Design review of the part built by this model. Coordinates are the model's own, in mm. A direction names the side the tool comes from. Round coordinates to 2 decimals unless told otherwise and drop trailing zeros. Order: outer loops, then holes, each group sorted by start corner. A loop starts at its lowest first (then second) coordinate and runs counter-clockwise, first axis right, second up. Notation, with made-up numbers: M -6.75,-39.75 L 29.25,-39.75 A19 ccw 29.25,-11.75 Z; hole C -21,14.25 d2. An arc over 180 degrees is marked long. Write each question's results on one line, items separated by ' | '. Start each with the question number.
Item 1: Take a section at A-A, the plane z = 0. Write out the cut boundary in (x, y), plus the area to 3 significant figures.
Item 2: Wall thickness on line 1 (X direction, y = -40.5, z = 6); line 2 (Z direction, x = 15, y = 37); line 3 (Y direction, x = 151, z = -5): over which ranges is each line inside the solid? List them lowest first. Write a range as [from, to].
Item 3: Machinability: for faces 1 (the flat face through (22, 42.2, 0.1)), 2 (the flat face through (74, 11, 7.5)), 3 (the flat face through (187, -11, -11)), 4 (the flat face through (107.186, 13.474, 0.105)), which of the approach directions +Z, -Z, +X, -X, +Y, -Y give a long, thin tool a straight path to every point of the face, cutting with its end or side? Answer none if there is none.
Item 4: Take a section at C-C, the plane x = 148.5. Write out the cut boundary in (y, z), plus the area to 3 significant figures.
Item 5: Take a section at B-B, the plane y = 0. Write out the cut boundary in (x, z), plus the area to 3 significant figures.
Item 6: Clearance check with flat-ended pins moving along their axes: pin 1 (4 mm diameter, centred on y = -5, z = 0, fed in from +X); pin 2 (4 mm diameter, centred on x = 56, z = -3, fed in from -Y); pin 3 (9 mm diameter, centred on y = 37, z = 0, fed in from -X); pin 4 (1 mm diameter, centred on x = 123.5, z = -4.5, fed in from -Y). State where each tip first meets the part, or that it passes through.
Item 7: The part is to be moulded in two halves that separate along Y. For faces 5 (the flat face through (22, -41, 3.4)), 6 (the cylindrical face through (195.163, -6.128, 0.154)), 7 (the flat face through (104.692, -8.598, 0.105)), 8 (the flat face through (104.692, 8.598, 0.105)), say which applies: +Y half, -Y half, draft (parallel to the pull), parting line (faces both ways), or undercut.
Item 8: Take a section at D-D, the plane y = 29. Write out the cut boundary in (x, z).
```python
from build123d import *

# Parameters (mm, degrees)
PAD_DEPTH          = 7.5
PAD001_DEPTH       = 17.5
PAD002_DEPTH       = 22
SKETCH_R           = 5
POCKET_DEPTH       = 22
POLARPATTERN_COUNT = 2
SKETCH004_R        = 16
PAD003_DEPTH       = 11
SKETCH005_R        = 11
POCKET001_DEPTH    = 22
CHAMFER_SIZE       = 1.5
CHAMFER001_SIZE    = 1.5


with BuildPart() as part:
    # CopySketch → Pad (new body, symmetric)
    with BuildSketch(Plane.XY):
        with BuildLine():
            Line((0, 31), (0, 37))
            Line((0, 37), (22, 37))
            Line((22, 37), (22, 31.4212968542))
            ThreePointArc((22, 31.4212968542), (37.2437089984, 20.6317995096), (55.3832021879, 16.1885232623))
            Line((55.3832021879, 16.1885232623), (160.4601470712, 10.6816739271))
            ThreePointArc((160.4601470712, 10.6816739271), (166.4509055525, 11.2749850989), (171.9937191701, 13.6241173914))
            ThreePointArc((171.9937191701, 13.6241173914), (164.3832021879, -3.37e-07), (171.993719744, -13.6241177448))
            ThreePointArc((171.993719744, -13.6241177448), (166.450905879, -11.2749851822), (160.4601470712, -10.6816739271))
            Line((55.3832021879, -16.1885232623), (160.4601470712, -10.6816739271))
            ThreePointArc((55.3832021879, -16.1885232623), (37.2437089984, -20.6317995096), (22, -31.4212968542))
            Line((22, -37), (22, -31.4212968542))
            Line((0, -37), (22, -37))
            Line((0, -31), (0, -37))
            ThreePointArc((0, -31), (31, 0), (0, 31))
        make_face()
        with BuildLine():
            ThreePointArc((154.7990604967, -5.9714971728), (161.3832021879, 0), (154.7990604967, 5.9714971728))
            Line((55.9676031362, 11.1510343764), (154.7990604967, 5.9714971728))
            ThreePointArc((55.9676031362, 11.1510343764), (44.2168647341, -1.26234e-05), (55.9676283484, -11.151033055))
            Line((55.9676283484, -11.151033055), (154.7990604967, -5.9714971728))
        make_face(mode=Mode.SUBTRACT)
    extrude(amount=PAD_DEPTH, both=True)

    # Sketch001 → Pad001 (join, symmetric)
    with BuildSketch(Plane.XY):
        with BuildLine():
            ThreePointArc((0, -25), (25, 0), (0, 25))
            Line((0, 31), (0, 25))
            ThreePointArc((0, -31), (31, 0), (0, 31))
            Line((0, -25), (0, -31))
        make_face()
    extrude(amount=PAD001_DEPTH, both=True)

    # Sketch003 → Pad002 (join)
    with BuildSketch(Plane.YZ):
        with BuildLine():
            ThreePointArc((37, -7.5), (44.5, 0), (37, 7.5))
            Line((37, 7.5), (37, -7.5))
        make_face()
        with BuildLine():
            ThreePointArc((-37, 7.5), (-44.5, 0), (-37, -7.5))
            Line((-37, 7.5), (-37, -7.5))
        make_face()
    extrude(amount=PAD002_DEPTH)

    # Sketch (on Face13 of Pad002) → Pocket (cut)
    with BuildSketch(Plane(origin=(0, 0, 0), x_dir=(0, -1, 0), z_dir=(-1, 0, 0))):
        with Locations((-37, 0)):
            Circle(SKETCH_R)
    pocket = extrude(amount=-POCKET_DEPTH, mode=Mode.SUBTRACT)

    # PolarPattern: Pocket ×2 about axis
    polarpattern_axis = Axis((0, 0, 0), (-1, 0, 0))
    for i in range(1, POLARPATTERN_COUNT):
        add(pocket.rotate(polarpattern_axis, i * 360 / POLARPATTERN_COUNT), mode=Mode.SUBTRACT)

    # Sketch004 → Pad003 (join, symmetric)
    with BuildSketch(Plane.XY):
        with Locations((180.383202, 0)):
            Circle(SKETCH004_R)
    extrude(amount=PAD003_DEPTH, both=True)

    # Sketch005 (on Face3 of Pad003) → Pocket001 (cut)
    with BuildSketch(Plane.XY.offset(11)):
        with Locations((180.383202, 0)):
            Circle(SKETCH005_R)
    extrude(amount=-POCKET001_DEPTH, mode=Mode.SUBTRACT)

    # Chamfer
    chamfer_edges = [part.edges().sort_by_distance(p)[0] for p in [
        (169.383202, 0, 11),
    ]]
    chamfer(chamfer_edges, length=CHAMFER_SIZE)

    # Chamfer001
    chamfer001_edges = [part.edges().sort_by_distance(p)[0] for p in [
        (169.383202, 0, -11),
    ]]
    chamfer(chamfer001_edges, length=CHAMFER001_SIZE)


solid = part.part
```
Results list:
1) outline: M 0,-44.5 L 22,-44.5 L 22,-42 L 0,-42 Z; M 0,-32 L 22,-32 L 22,-31.42 A50 cw 55.38,-16.19 L 160.46,-10.68 A20 cw 171.99,-13.62 A16 ccw long 171.99,13.62 A20 cw 160.46,10.68 L 55.38,16.19 A50 cw 22,31.42 L 22,32 L 0,32 L 0,25 A25 cw 0,-25 Z; M 0,42 L 22,42 L 22,44.5 L 0,44.5 Z; hole M 55.97,-11.15 L 154.8,-5.97 A6 ccw long 154.8,5.97 L 55.97,11.15 A11.17 ccw long Z; hole C 180.38,0 d22 | area: 3,360 mm²
2) line 1: [0, 22] | line 2: [-7.5, -5], [5, 7.5] | line 3: [-11.18, -6.17], [6.17, 11.18]
3) face 1: +Z, -Z, +X, +Y | face 2: +Z | face 3: -Z, +X, +Y, -Y | face 4: +Z, -Z, +Y
4) outline: M -11.31,-7.5 L -6.3,-7.5 L -6.3,7.5 L -11.31,7.5 Z; M 6.3,-7.5 L 11.31,-7.5 L 11.31,7.5 L 6.3,7.5 Z | area: 150 mm²
5) outline: M 25,-17.5 L 31,-17.5 L 31,-7.5 L 44.22,-7.5 L 44.22,7.5 L 31,7.5 L 31,17.5 L 25,17.5 Z; M 161.38,-7.5 L 164.38,-7.5 L 164.38,-11 L 167.88,-11 L 169.38,-9.5 L 169.38,9.5 L 167.88,11 L 164.38,11 L 164.38,7.5 L 161.38,7.5 Z; M 191.38,-9.5 L 192.88,-11 L 196.38,-11 L 196.38,11 L 192.88,11 L 191.38,9.5 Z | area: 669 mm²
6) pin 1: x = 196.1 | pin 2: y = -16.28 | pin 3: through | pin 4: y = -12.64
7) face 5: draft | face 6: parting line | face 7: undercut | face 8: undercut
8) outline: M 0,-17.5 L 10.95,-17.5 L 10.95,-7.5 L 24.5,-7.5 L 24.5,7.5 L 10.95,7.5 L 10.95,17.5 L 0,17.5 Z
